Geometry: final body of the model. Coordinates: model frame, mm. Face numbers are marked on the shaded views. A direction names the side the tool comes from. Coordinates: 2 decimals unless noted, no trailing zeros. Write each loop counter-clockwise with the first axis right and the second up, starting at its lowest first coordinate (ties: lowest second). Pieces come first, ordered by that corner, then holes.
from build123d import *

# Parameters (mm, degrees)
SKETCH1_W           = 30
SKETCH1_H           = 38.7
BOSS_EXTRUDE1_DEPTH = 3
BOSS_EXTRUDE2_DEPTH = 4.3
FILLET1_R           = 1
SKETCH3_R           = 1.1
CUT_EXTRUDE1_DEPTH  = 25.857845844
BOSS_EXTRUDE3_START = 2.7
SKETCH4_R           = 2.1
SKETCH4_R_2         = 1.1
BOSS_EXTRUDE3_DEPTH = 2.7
BOSS_EXTRUDE4_START = 5
BOSS_EXTRUDE4_DEPTH = 2.3
FILLET2_R           = 5


with BuildPart() as part:
    # Sketch1 → Boss-Extrude1 (new body)
    with BuildSketch(Plane(origin=(0, 0, 0), x_dir=(1, 0, 0), z_dir=(0, 1, 0))):
        Rectangle(SKETCH1_W, SKETCH1_H)
    extrude(amount=BOSS_EXTRUDE1_DEPTH)

    # Sketch2 → Boss-Extrude2 (add)
    with BuildSketch(Plane(origin=(0, 3, 0), x_dir=(1, 0, 0), z_dir=(0, 1, 0))):
        Polygon((-13, 17.35), (-13, -19.35), (-15, -19.35), (-15, 19.35), (15, 19.35), (15, -19.35), (13, -19.35), (13, 17.35), align=None)
    extrude(amount=BOSS_EXTRUDE2_DEPTH)

    # Fillet1
    fillet1_edges = [part.edges().sort_by_distance(p)[0] for p in [
        (-13, 5.15, -17.35),
        (13, 5.15, -17.35),
    ]]
    fillet(fillet1_edges, radius=FILLET1_R)

    # Sketch3 → Cut-Extrude1 (cut, through all)
    with BuildSketch(Plane(origin=(0, 3, 0), x_dir=(1, 0, 0), z_dir=(0, 1, 0))):
        with Locations(Location((-10, 14.57312599, 0), (0, 0, 270))):
            Circle(SKETCH3_R)
        with Locations(Location((10, 14.57312599, 0), (0, 0, 270))):
            Circle(SKETCH3_R)
        with Locations(Location((-10, -5.42687401, 0), (0, 0, 270))):
            Circle(SKETCH3_R)
        with Locations(Location((10.317528275, -5.42687401, 0), (0, 0, 270))):
            Circle(SKETCH3_R)
    extrude(amount=-CUT_EXTRUDE1_DEPTH, mode=Mode.SUBTRACT)

    # Sketch4 → Boss-Extrude3 (add)
    # profile 1 of 4: a face of its own
    with BuildSketch(Plane(origin=(0, 3, 0), x_dir=(1, 0, 0), z_dir=(0, 1, 0)).offset(BOSS_EXTRUDE3_START)):
        with Locations(Location((-10, 14.57312599, 0), (0, 0, 270))):
            Circle(SKETCH4_R)
        with Locations(Location((-10, 14.57312599, 0), (0, 0, 270))):
            Circle(SKETCH4_R_2, mode=Mode.SUBTRACT)
    # profile 2 of 4: a face of its own
    with BuildSketch(Plane(origin=(0, 3, 0), x_dir=(1, 0, 0), z_dir=(0, 1, 0)).offset(BOSS_EXTRUDE3_START)):
        with Locations(Location((10, 14.57312599, 0), (0, 0, 270))):
            Circle(SKETCH4_R)
        with Locations(Location((10, 14.57312599, 0), (0, 0, 270))):
            Circle(SKETCH4_R_2, mode=Mode.SUBTRACT)
    # profile 3 of 4: a face of its own
    with BuildSketch(Plane(origin=(0, 3, 0), x_dir=(1, 0, 0), z_dir=(0, 1, 0)).offset(BOSS_EXTRUDE3_START)):
        with Locations(Location((10.317528275, -5.42687401, 0), (0, 0, 270))):
            Circle(SKETCH4_R)
        with Locations(Location((10.317528275, -5.42687401, 0), (0, 0, 270))):
            Circle(SKETCH4_R_2, mode=Mode.SUBTRACT)
    # profile 4 of 4: a face of its own
    with BuildSketch(Plane(origin=(0, 3, 0), x_dir=(1, 0, 0), z_dir=(0, 1, 0)).offset(BOSS_EXTRUDE3_START)):
        with Locations(Location((-10, -5.42687401, 0), (0, 0, 270))):
            Circle(SKETCH4_R)
        with Locations(Location((-10, -5.42687401, 0), (0, 0, 270))):
            Circle(SKETCH4_R_2, mode=Mode.SUBTRACT)
    extrude(amount=-BOSS_EXTRUDE3_DEPTH)

    # Sketch5 → Boss-Extrude4 (add)
    with BuildSketch(Plane(origin=(0, 0, 0), x_dir=(1, 0, 0), z_dir=(0, 1, 0)).offset(BOSS_EXTRUDE4_START)):
        Polygon((-21, 25.35), (21, 25.35), (21, -19.35), (15, -19.35), (15, 19.35), (-15, 19.35), (-15, -19.35), (-21, -19.35), align=None)
    extrude(amount=BOSS_EXTRUDE4_DEPTH)

    # Fillet2
    fillet2_edges = [part.edges().sort_by_distance(p)[0] for p in [
        (-21, 6.15, -25.35),
        (21, 6.15, -25.35),
    ]]
    fillet(fillet2_edges, radius=FILLET2_R)


solid = part.part
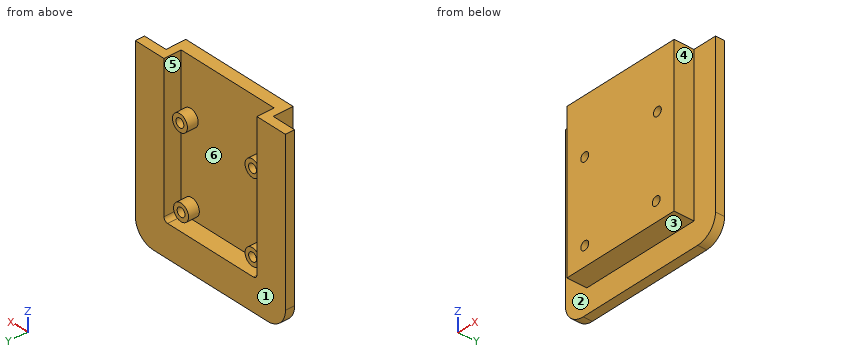
Item 1: Set-up query: the marked faces 1 and 2. Return all of +Z, -Z, +X, -X, +Y, -Y with unobstructed straight access to the full face (end or side cutting, diameter ignored); none if empty.
Derived:
face 1: +Z, -Z, +X, -X, +Y
face 2: -Z, -Y
Item 2: Section A-A, the plane y = 3.5. State how many separate pieces and enclosed holes the cut face has, plus the area to 3 significant figures.
Derived:
separate pieces: 5
enclosed holes: 4
area: 247 mm2
Item 3: Section B-B, the plane z = 11. Output: boundary loops of the cut face in (x, y), plus the area to 3 significant figures.
Derived:
outline: (-21, 5) - (-15, 5) - (-15, 0) - (15, 0) - (15, 5) - (21, 5) - (21, 7.3) - (13, 7.3) - (13, 3) - (-13, 3) - (-13, 7.3) - (-21, 7.3) - close
area: 135 mm2
Item 4: Pull-direction query (X, two-part tool) for the marked faces 3, 4, 5 and 6; classes: released by +X, released by -X, zero draft, split by the parting line, or undercut.
Derived:
face 3: zero draft
face 4: released by +X
face 5: undercut
face 6: undercut
Item 5: Section C-C, the plane x = -10. Output: boundary loops of the cut face in (y, z), plus the area to 3 significant figures.
Derived:
outline: (0, -19.35) - (5, -19.35) - (5, -25.35) - (7.3, -25.35) - (7.3, -17.35) - (3, -17.35) - (3, -16.67) - (5.7, -16.67) - (5.7, -15.67) - (0, -15.67) - close; (0, -13.47) - (5.7, -13.47) - (5.7, -12.47) - (3, -12.47) - (3, 3.33) - (5.7, 3.33) - (5.7, 4.33) - (0, 4.33) - close; (0, 6.53) - (5.7, 6.53) - (5.7, 7.53) - (3, 7.53) - (3, 19.35) - (0, 19.35) - close
area: 136 mm2
Item 6: Pin query (flat end, axial travel): pin 1 (4.5 mm diameter, centred on x = 10.5, z = -14, fed in from +Y); pin 2 (1.5 mm diameter, centred on x = -5.5, y = 2.5, fed in from -Z); pin 3 (1.3 mm diameter, centred on x = -0.5, y = 5.5, fed in from +Z); pin 4 (3.5 mm diameter, centred on x = -10, z = 5.43, fed in from -Y). Return the tip coordinate at first contact, or that it passes through.
Derived:
pin 1: stops at y = 5.7
pin 2: stops at z = -19.35
pin 3: stops at z = -17.35
pin 4: stops at y = 0
Item 7: Section D-D, the plane y = 6.25. Output: boundary loops of the cut face in (x, z), plus the area to 3 significant figures.
Derived:
outline: (-21, -20.35) arc R5 ccw to (-16, -25.35) - (16, -25.35) arc R5 ccw to (21, -20.35) - (21, 19.35) - (13, 19.35) - (13, -16.35) arc R1 cw to (12, -17.35) - (-12, -17.35) arc R1 cw to (-13, -16.35) - (-13, 19.35) - (-21, 19.35) - close
area: 913 mm2
Item 8: Material intervals for probe 1 along X at (y, z) = (3.5, -0.5); probe 2 along X at (y, z) = (6.25, 15); probe 3 along Y at (x, z) = (-4, 15), sorted ascending.
Derived:
probe 1: x = -15 to -13, 13 to 15
probe 2: x = -21 to -13, 13 to 21
probe 3: y = 0 to 3
